```python
from build123d import *

# Parameters (mm, degrees)
F0_W          = 35
F0_H          = 18
F1_DEPTH      = 20
F2_W          = 30
F2_H          = 23.709095493
F3_DEPTH      = 15
F5_DEPTH      = 32.5
F6_T1_DEPTH   = 53.9336597593
F7_R          = 2
F10_DEPTH     = 25
F11_R         = 5
F12_W         = 16
F12_H         = 17.5
F13_DEPTH     = 1.5
F14_T4_DEPTH  = 26.4267855357
F14_T9_DEPTH  = 26.4267855357
F14_T11_DEPTH = 28
F14_T13_DEPTH = 28
F15_R         = 1.2
F16_DEPTH     = 3.0010001


# Not quite as in the source:
# - a fillet or chamfer that OpenCascade refuses, or shapes differently, is made with other operations: its cross-section is extruded or revolved along the edge and cut away or added


with BuildPart() as f1:
    # F0 (on Front) → F1 (new body)
    with BuildSketch(Plane.XZ):
        with Locations((0, 9)):
            Rectangle(F0_W, F0_H)
    extrude(amount=F1_DEPTH)

    # F2 (on face) → F3 (cut)
    with BuildSketch(Plane.XY.offset(18)):
        with Locations((0, -14.3545477465)):
            Rectangle(F2_W, F2_H)
    extrude(amount=-F3_DEPTH, mode=Mode.SUBTRACT)

    # F4 (on face) → F5 (cut, symmetric)
    with BuildSketch(Plane(origin=(15, 0, 0), x_dir=(0, -1, 0), z_dir=(-1, 0, 0))):
        Polygon((20, 18), (2.5, 18), (20, 3), align=None)
    extrude(amount=F5_DEPTH, both=True, mode=Mode.SUBTRACT)

    # F6: chamfer of 10 on 2 edges, made by hand

    # F6_s2 → F6_t1 (cut)
    with BuildSketch(Plane.XZ.offset(-25.7168298797)):
        Polygon((17.5, 8), (7.5, 18), (17.5, 18), align=None)
        Polygon((-7.5, 18), (-17.5, 8), (-17.5, 18), align=None)
    extrude(amount=F6_T1_DEPTH, mode=Mode.SUBTRACT)

    # F7
    f7_edges = [f1.edges().sort_by_distance(p)[0] for p in [
        (-15, -2.5, 6.75),
        (15, -2.5, 6.75),
        (-15, -11.25, 3),
        (15, -11.25, 3),
    ]]
    fillet(f7_edges, radius=F7_R)

    # F8 (on face) → F10 (cut)
    with BuildSketch(Plane(origin=(0, 0, 0), x_dir=(-1, 0, 0), z_dir=(0, 1, 0))):
        with BuildLine():
            Line((-1.409787218, 5.65), (1.409787218, 5.65))
            ThreePointArc((1.409787218, 5.65), (4.0923866141, 9.2502565294), (1.8674849397, 13.15))
            Line((1.8674849397, 13.15), (0.9, 13.15))
            Line((0.9, 13.15), (0.9, 14.5))
            Line((0.9, 14.5), (-0.9, 14.5))
            Line((-0.9, 14.5), (-0.9, 13.15))
            Line((-0.9, 13.15), (-1.8674849397, 13.15))
            ThreePointArc((-1.8674849397, 13.15), (-4.0923866141, 9.2502565294), (-1.409787218, 5.65))
        make_face()
    extrude(amount=-F10_DEPTH, mode=Mode.SUBTRACT)

    # F11
    f11_edges = [f1.edges().sort_by_distance(p)[0] for p in [
        (7.5, -1.25, 18),
        (-7.5, -1.25, 18),
        (17.5, 0, 4),
        (-17.5, 0, 4),
    ]]
    fillet(f11_edges, radius=F11_R)

    # F12 (on face) → F13 (cut)
    with BuildSketch(Plane.XY.offset(3)):
        with Locations((0, -11.25)):
            Rectangle(F12_W, F12_H)
    extrude(amount=-F13_DEPTH, mode=Mode.SUBTRACT)

    # F14: fillet of radius 5 on 4 edges, made by hand


with BuildPart() as f14_tool2:
    # F14_s3 → F14_t4 (new body)
    with BuildSketch(Plane.XZ.offset(20)):
        with BuildLine():
            ThreePointArc((8, 3), (6.3657774588, 1.8902277714), (4.4292857857, 1.5))
            Line((4.4292857857, 1.5), (8, 1.5))
            Line((8, 1.5), (8, 3))
        make_face()
    extrude(amount=-F14_T4_DEPTH)

    split(bisect_by=Plane.XZ, keep=Keep.TOP)


with BuildPart() as f1_1:
    add(f1.part)

    # F14_t1: union F14_tool2
    add(f14_tool2.part)


with BuildPart() as f14_tool7:
    # F14_s8 → F14_t9 (new body)
    with BuildSketch(Plane.XZ.offset(-6.4267855357)):
        with BuildLine():
            ThreePointArc((-8, 3), (-6.3657774588, 1.8902277714), (-4.4292857857, 1.5))
            Line((-4.4292857857, 1.5), (-8, 1.5))
            Line((-8, 1.5), (-8, 3))
        make_face()
    extrude(amount=F14_T9_DEPTH)

    split(bisect_by=Plane.XZ, keep=Keep.TOP)


with BuildPart() as f1_2:
    add(f1_1.part)

    # F14_t6: union F14_tool7
    add(f14_tool7.part)

    # F14_s12 → F14_t11 (cut)
    with BuildSketch(Plane.XY.offset(-12.5)):
        with BuildLine():
            ThreePointArc((17.5, -15), (16.0355339059, -18.5355339059), (12.5, -20))
            Line((12.5, -20), (17.5, -20))
            Line((17.5, -20), (17.5, -15))
        make_face()
    extrude(amount=F14_T11_DEPTH, mode=Mode.SUBTRACT)

    # F14_s14 → F14_t13 (cut)
    with BuildSketch(Plane.XY.offset(-12.5)):
        with BuildLine():
            ThreePointArc((-17.5, -15), (-16.0355339059, -18.5355339059), (-12.5, -20))
            Line((-12.5, -20), (-17.5, -20))
            Line((-17.5, -20), (-17.5, -15))
        make_face()
    extrude(amount=F14_T13_DEPTH, mode=Mode.SUBTRACT)

    # F15 (on face) → F16 (cut, through all)
    with BuildSketch(Plane.XY.offset(3)):
        with Locations((-10.5, -10.5)):
            Circle(F15_R)
        with BuildLine():
            ThreePointArc((11.7, -10.5), (10.5, -9.3), (9.3, -10.5))
            ThreePointArc((9.3, -10.5), (10.5, -11.7), (11.7, -10.5))
        make_face()
    extrude(amount=-F16_DEPTH, mode=Mode.SUBTRACT)


solid = f1_2.part
```
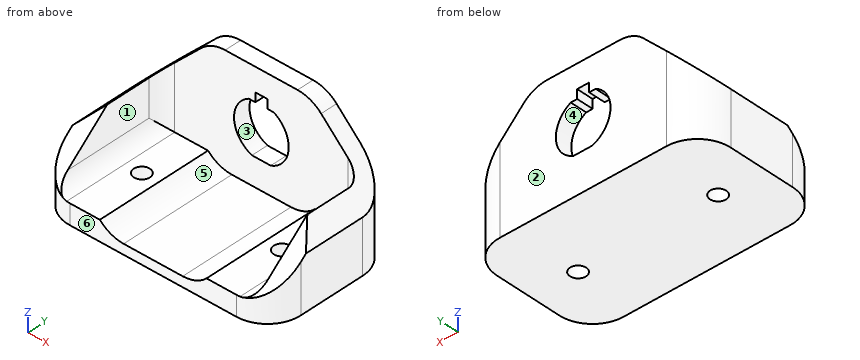
Input: part model. Units: mm. Frame: model coordinates. Face numbers are marked on the shaded views. A direction names the side the tool comes from. Round coordinates to 2 decimals unless told otherwise and drop trailing zeros. Write each loop counter-clockwise with the first axis right and the second up, starting at its lowest first coordinate (ties: lowest second). Pieces come first, ordered by that corner, then holes. Notation, with made-up numbers: (7, 32) -> (56, 32) arc R12 cw to (56, 45) -> close; hole circle Ø9 at (-22.5, 29). An arc over 180 degrees is marked (long way). Answer as CSV lines item,"result".
1. Mould query, pull axis Z, two halves, no side actions, for the marked faces 4, 5 and 6. Classes: +Z half, -Z half, draft (parallel to the pull), parting line (faces both ways), or undercut.
Geometry says:
face 4,"undercut"
face 5,"+Z half"
face 6,"draft"
2. Section D-D (y = -12.5). Return the cut outline in (x, z), plus the area to 3 significant figures.
Geometry says:
outline,"(-17.5, 0) -> (17.5, 0) -> (17.5, 8) -> (16.07, 9.43) -> (15, 9.43) -> (15, 5) arc R2 cw to (13, 3) -> (8, 3) arc R5 cw to (4.43, 1.5) -> (-4.43, 1.5) arc R5 cw to (-8, 3) -> (-13, 3) arc R2 cw to (-15, 5) -> (-15, 9.43) -> (-16.07, 9.43) -> (-17.5, 8) -> close"
area,"116 mm^2"
3. Contact query for flat-ended pins moving along their axis: P1, Ø1.1, axis at y = -2, z = 14, coming from the -X side; P2, Ø2, axis at x = 11.5, z = 9.5, coming from the -Y side; P3, Ø1.5, axis at y = -1.5, z = 14, coming from the +X side; P4, Ø4, axis at x = 13.5, z = 15, coming from the +Y side. Output: stop coordinate, or through.
Geometry says:
P1,"stops at x = -12.05"
P2,"stops at y = -2.5"
P3,"stops at x = 12.25"
P4,"passes through"
4. Reachability of the marked faces 1, 2 and 3 from +Z, -Z, +X, -X, +Y, -Y: full face, straight path, thin tool, end or side. Return the list, or none.
Geometry says:
face 1,"+Z, -Y"
face 2,"+Z, -Z, +X, -X, +Y"
face 3,"+Y, -Y"
5. Ray query, L1, parallel to Y at x = -10.5, z = 1; L2, parallel to X at y = -7.75, z = 6.5; L3, parallel to Y at x = 4, z = 1.75. Return the intervals inside material, ascending. Write a range as [from, to].
Geometry says:
L1,"y = [-20, -11.7], [-9.3, 0]"
L2,"x = [-17.5, -15], [15, 17.5]"
L3,"y = [-2.5, 0]"
6. Section C-C (y = -18.5). Return the cut outline in (x, z), plus the area to 3 significant figures.
Geometry says:
outline,"(-16.07, 0) -> (16.07, 0) -> (16.07, 4.29) -> (14.87, 4.29) arc R2 cw to (13, 3) -> (8, 3) arc R5 cw to (4.43, 1.5) -> (-4.43, 1.5) arc R5 cw to (-8, 3) -> (-13, 3) arc R2 cw to (-14.87, 4.29) -> (-16.07, 4.29) -> close"
area,"80.2 mm^2"
7. Section B-B (y = -9.75). Return the cut outline in (x, z).
Geometry says:
outline,"(-17.5, 0) -> (-11.44, 0) -> (-11.44, 3) -> (-13, 3) arc R2 cw to (-15, 5) -> (-15, 10.5) -> (-17.5, 8) -> close; (-9.56, 0) -> (9.56, 0) -> (9.56, 3) -> (8, 3) arc R5 cw to (4.43, 1.5) -> (-4.43, 1.5) arc R5 cw to (-8, 3) -> (-9.56, 3) -> close; (11.44, 0) -> (17.5, 0) -> (17.5, 8) -> (15, 10.5) -> (15, 5) arc R2 cw to (13, 3) -> (11.44, 3) -> close"
8. Section A-A (x = 10.5). Return the cut outline in (y, z), plus the area to 3 significant figures.
Geometry says:
outline,"(-20, 0) -> (-11.7, 0) -> (-11.7, 3) -> (-20, 3) -> close; (-9.3, 0) -> (0, 0) -> (0, 15) -> (-2.5, 15) -> (-2.5, 3) -> (-9.3, 3) -> close"
area,"82.8 mm^2"
